Verification items for the finished model (mm, model axes). A direction names the side the tool comes from. Give positions to 0.01 mm unless a question says otherwise; leave off trailing zeros. Write each loop counter-clockwise with the first axis right and the second up, starting at its lowest first coordinate (ties: lowest second). Pieces come first, ordered by that corner, then holes. Notation, with made-up numbers: M 50,-2 L 109,-2 A29 cw 109,30 Z; hole C 49.5,30 d2. An arc over 180 degrees is marked long. Answer as a JSON object with one key per item and string values.
Autodesk Inventor part; units mm, degrees
ref_plane "YZ Plane" through (0, 0, 0) normal (1, 0, 0) x (0, 1, 0)
ref_plane "XZ Plane" through (0, 0, 0) normal (0, 1, 0) x (-1, 0, 0)
ref_plane "XY Plane" through (0, 0, 0) normal (0, 0, 1) x (1, 0, 0)
sketch "Skizze1" plane through (0, 0, 0) normal (0, 1, 0) x (-1, 0, 0)
  line L0 (0, 0) -> (105, 0)
  line L1 (105, 0) -> (105, -105)
  line L2 (105, -105) -> (0, -105)
  line L3 (0, -105) -> (0, 0)
  line L4 (0, -105) -> (93, -105)
  line L5 (93, -105) -> (93, 0)
  line L6 (93, 0) -> (0, 0)
  line L7 (0, 0) -> (0, -105)
  dimension "d0" = 105
  dimension "d1" = 105
  dimension "d2" = 93
extrude "Extrusion1" add sketch "Skizze1" along normal blind 45 contours L0 L5 L2 L3
sketch "Skizze2" plane through (0, 0, 0) normal (0, -1, 0) x (1, 0, 0)
  line L0 (0, -105) -> (-93, -105)
  line L1 (-93, -105) -> (12, -105)
  line L2 (12, -105) -> (12, 0)
  line L3 (12, 0) -> (-93, 0)
  line L4 (-93, 0) -> (-93, -105)
  line L5 (-93, -105) -> (-93, 0)
  line L6 (12, -105) -> (-93, -105)
  line L7 (-93, -105) -> (-93, -95)
  line L8 (-93, -95) -> (12, -95)
  line L9 (12, -95) -> (12, -105)
  line L10 (12, 0) -> (-93, 0)
  line L11 (-93, 0) -> (-93, -10)
  line L12 (-93, -10) -> (12, -10)
  line L13 (12, -10) -> (12, 0)
  point P0 (0, 0)
  point P1 (12, -10)
  point P2 (12, -95)
  dimension "d5" = 105
  dimension "d6" = 10
  dimension "d7" = 10
extrude "Extrusion2" add sketch "Skizze2" along normal blind 20 contours L0 L4 L8 L2 L1 | L4 L3 L2 L12
sketch "Skizze3" plane through (0, 0, 0) normal (0, 1, 0) x (1, 0, 0)
  line L0 (-93, 0) -> (0, 0)
  line L1 (0, 105) -> (12, 105)
  line L2 (0, 0) -> (12, 0)
  line L3 (12, 0) -> (12, 105)
  line L4 (12, 105) -> (0, 105)
  line L5 (0, 105) -> (0, 0)
extrude "Extrusion3" add sketch "Skizze3" along normal blind 15
sketch "Skizze4" plane through (0, 45, -105) normal (0, 0, -1) x (-1, 0, 0)
  line L0 (93, -65) -> (93, 0)
  line L1 (0, 0) -> (93, 0)
  line L2 (0, -30) -> (0, 0)
  line L3 (-12, -30) -> (0, -30)
  line L4 (-12, -30) -> (-12, -65)
  line L5 (93, -65) -> (-12, -65)
  line L6 (3, -3) -> (90, -3)
  line L7 (90, -3) -> (90, -26)
  line L8 (90, -26) -> (3, -26)
  line L9 (3, -26) -> (3, -3)
  point P0 (0, -45)
  point P1 (46.5, -3)
  point P2 (46.5, 0)
  dimension "d12" = 3
  dimension "d13" = 3
  dimension "d14" = 23
extrude "Extrusion4" cut sketch "Skizze4" against normal through all contours L6 L7 L8 L9
equation "\"d0\" = base_breite"
equation "\"d1\" = base_tiefe"
equation "\"d2\" = koerper_breite"
equation "\"d3\" = hoehe - fuss_höhe"
equation "\"d5\" = base_breite"
equation "\"d6\" = fuss_breite"
equation "\"d7\" = fuss_breite"
equation "\"d8\" = fuss_höhe"
equation "\"d10\" = PCI_hoehe"
equation "\"d12\" = koerper_wandstaerke"
equation "\"d13\" = koerper_wandstaerke"
equation "\"d14\" = kuehlöffnung"
equation "\"base_breite\" = 105"
equation "\"base_tiefe\" = 105"
equation "\"fuss_breite\" = 10"
equation "\"koerper_breite\" = 93"
equation "\"koerper_tiefe\" = 105"
equation "\"fuss_höhe\" = 20"
equation "\"hoehe\" = 65"
equation "\"PCI_hoehe\" = 15"
equation "\"koerper_wandstaerke\" = 3"
equation "\"kuehlöffnung\" = 23"
properties part number "jetson_dummy"
1) Section check B-B on x = -35. Record the boundary of the cut face in (y, z), and give its area (3 significant figures).
Completed:
{"outline": "M -20,-105 L 19,-105 L 19,0 L -20,0 L -20,-10 L 0,-10 L 0,-95 L -20,-95 Z; M 42,-105 L 45,-105 L 45,0 L 42,0 Z", "area": "2,710 mm2"}
2) Section check C-C on z = -59.5. Record the boundary of the cut face in (x, y).
Completed:
{"outline": "M -93,0 L 12,0 L 12,15 L 0,15 L 0,45 L -93,45 Z; hole M -90,19 L -3,19 L -3,42 L -90,42 Z"}
3) Go/stop test with flat-tipped pins: pin 1 (11.5 mm diameter, centred on y = 36, z = -60.5, fed in from +X); pin 2 (10 mm diameter, centred on y = -1, z = -85, fed in from +X); pin 3 (6 mm diameter, centred on x = 5.5, z = -60.5, fed in from +Y). Record where each tip stops, or that it passes through.
Completed:
{"pin 1": "stops at x = 0", "pin 2": "stops at x = 12", "pin 3": "stops at y = 15"}
4) Section check D-D on y = 39.5. Record the boundary of the cut face in (x, z), and give its area (3 significant figures).
Completed:
{"outline": "M -93,-105 L -90,-105 L -90,0 L -93,0 Z; M -3,-105 L 0,-105 L 0,0 L -3,0 Z", "area": "630 mm2"}
5) Thickness scan on L1, parallel to Y at x = -15, z = -19; L2, parallel to Y at x = -84, z = -9.5; L3, parallel to X at y = 26, z = -88. Record the ranges inside material, lowest first.
Completed:
{"L1": "y = 0 to 19, 42 to 45", "L2": "y = -20 to 19, 42 to 45", "L3": "x = -93 to -90, -3 to 0"}
6) Release check for a two-part mould opening along X. For faces 4 (the face through (-3, 30, -53)), 5 (the face through (-41, -20, -100)), 6 (the face through (-93, 19, -53)) record: pulls with the +X half, pulls with the -X half, needs draft (parallel to the pull), parting line crosses it, or undercut.
Completed:
{"face 4": "undercut", "face 5": "needs draft", "face 6": "pulls with the -X half"}
7) Access from +Z, -Z, +X, -X, +Y, -Y to the whole of each face (thin tool, end or side, straight path). Record for faces 1 (the face through (-46, 42, -53)), 2 (the face through (-41, -10, -10)), 3 (the face through (6, 15, -53)).
Completed:
{"face 1": "+Z, -Z", "face 2": "+X, -X, -Y", "face 3": "+Z, -Z, +X, +Y"}
8) Section check A-A on y = -12. Record the boundary of the cut face in (x, z).
Completed:
{"outline": "M -93,-105 L 12,-105 L 12,-95 L -93,-95 Z; M -93,-10 L 12,-10 L 12,0 L -93,0 Z"}
